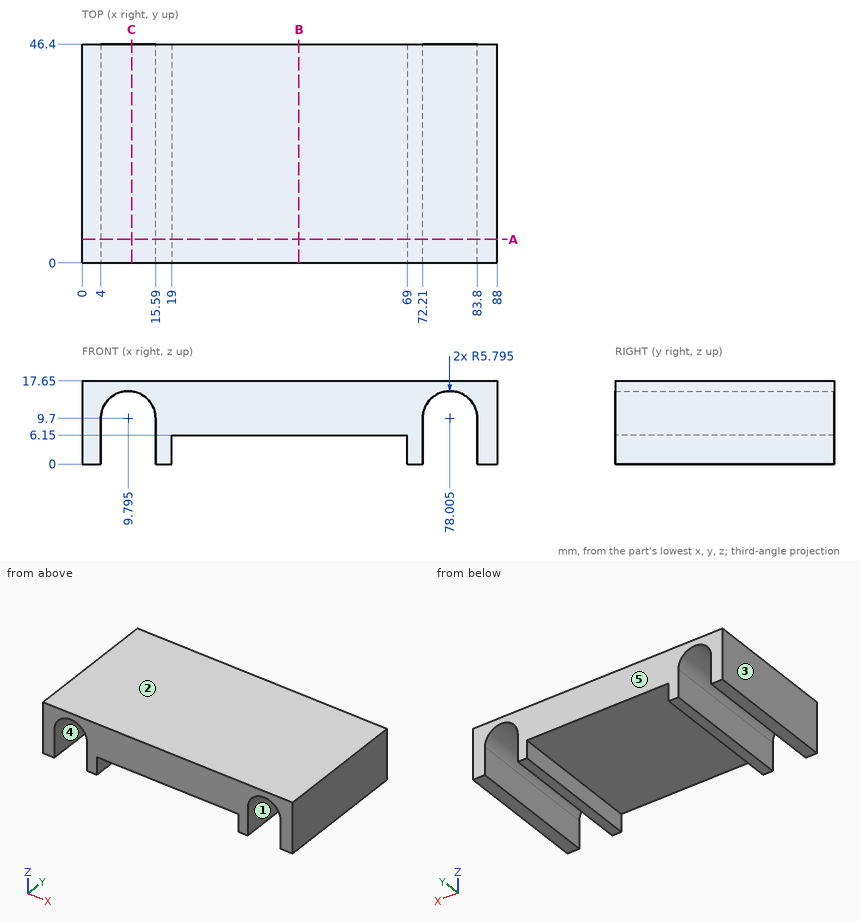
The figure shows three views and two pictorial views of one solid part (mm, origin at its lowest corner). Answer the questions. A direction names the side the tool comes from. Round coordinates to 2 decimals unless told otherwise and drop trailing zeros. Order: outer loops, then holes, each group sorted by start corner. A loop starts at its lowest first (then second) coordinate and runs counter-clockwise, first axis right, second up. Notation, with made-up numbers: (-12.5, 4.25) -> (31.5, 4.25) arc R28 ccw to (31.5, 24.25) -> close; hole circle Ø6 at (-39, 5). An arc over 180 degrees is marked (long way). Put each result on its own line as item: value.
Q1. Consider line 1 along X through (y, z) = (13, 5); line 2 along X through (y, z) = (27, 11); line 3 along X through (y, z) = (28.5, 12.5). Determine where each line is inside the solid, lowest interval first.
Results list:
line 1: 0 to 4, 15.59 to 19, 69 to 72.21, 83.8 to 88
line 2: 0 to 4.15, 15.44 to 72.36, 83.65 to 88
line 3: 0 to 4.72, 14.87 to 72.93, 83.08 to 88
Q2. Each of these flat-tipped pins is pushed along its axis until it touches: P1, Ø10, axis at x = 12, z = 3.5, coming from the +Y side; P2, Ø1.5, axis at x = 56.5, y = 12, coming from the -Z side. Where does it stop, or does it pass through?
Results list:
P1: y = 46.4
P2: z = 6.15
Q3. Section C-C, the plane x = 10.5 is taken. Write down the section's boundary in (y, z).
Results list:
outline: (0, 15.45) -> (46.4, 15.45) -> (46.4, 17.65) -> (0, 17.65) -> close
Q4. Which of the six approach directions +Z, -Z, +X, -X, +Y, -Y give full straight-line access (tool end or side, diameter ignored) to the marked faces 4 and 5?
Results list:
face 4: -Z, +Y, -Y
face 5: +Z, -Z, +X, -X, +Y
Q5. Section B-B, the plane x = 46 is taken. Write down the section's boundary in (y, z).
Results list:
outline: (0, 6.15) -> (46.4, 6.15) -> (46.4, 17.65) -> (0, 17.65) -> close
Q6. Section A-A, the plane y = 5 is taken. Write down the section's boundary in (x, z) (3 decimals).
Results list:
outline: (0, 0) -> (4, 0) -> (4, 9.7) arc R5.795 cw to (15.59, 9.7) -> (15.59, 0) -> (19, 0) -> (19, 6.15) -> (69, 6.15) -> (69, 0) -> (72.21, 0) -> (72.21, 9.7) arc R5.795 cw to (83.8, 9.7) -> (83.8, 0) -> (88, 0) -> (88, 17.65) -> (0, 17.65) -> close
Q7. Determine the mould class of the marked faces 1, 2 and 3 for opening direction X: pulls with the +X half, pulls with the -X half, needs draft (parallel to the pull), parting line crosses it, or undercut.
Results list:
face 1: undercut
face 2: needs draft
face 3: pulls with the -X half
